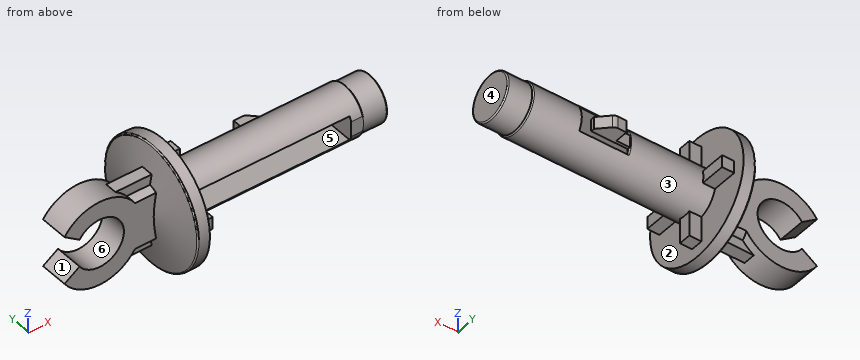
```python
from build123d import *

# Parameters (mm, degrees)
SCHIZZO1_R                    = 2
ESTRUSIONE_ESTRUSIONE1_DEPTH  = 17
SCHIZZO2_OUTSIDE_W            = 9.584
SCHIZZO2_OUTSIDE_H            = 9.584
SCHIZZO2_OUTSIDE_R            = 1.9
TAGLIO_ESTRUSIONE1_DEPTH      = 2
SCHIZZO6_W                    = 15
SCHIZZO6_H                    = 4
TAGLIO_ESTRUSIONE3_DEPTH      = 0.1
TAGLIO_ESTRUSIONE4_DEPTH      = 1.7
TAGLIO_ESTRUSIONE4_DEPTH_BACK = 18.23368794
SCHIZZO5_W                    = 13
SCHIZZO5_H                    = 2
SCHIZZO7_W                    = 4
SCHIZZO7_H                    = 2
TAGLIO_ESTRUSIONE5_DEPTH      = 18.555910686
ESTRUSIONE_ESTRUSIONE2_DEPTH  = 0.5
TAGLIO_ESTRUSIONE6_DEPTH      = 0.07
ESTRUSIONE_ESTRUSIONE4_DEPTH  = 0.5
ESTRUSIONE_ESTRUSIONE5_DEPTH  = 0.5
SCHIZZO20_R                   = 5
ESTRUSIONE_ESTRUSIONE6_DEPTH  = 1
SCHIZZO23_R                   = 2.25
ESTRUSIONE_ESTRUSIONE7_DEPTH  = 3
ESTRUSIONE_ESTRUSIONE10_DEPTH = 1.15
ESTRUSIONE_ESTRUSIONE8_DEPTH  = 0.5
SCHIZZO35_W                   = 3
SCHIZZO35_H                   = 3.867815922
TAGLIO_ESTRUSIONE7_DEPTH      = 1.3
RACCORDO22_R                  = 0.5
RACCORDO23_R                  = 0.1
RACCORDO24_R                  = 0.1
RACCORDO25_R                  = 0.1
RACCORDO28_R                  = 0.1


# Some blends are built 0.0001 mm under size
with BuildPart() as part:
    # Schizzo1 → Estrusione-Estrusione1 (new body)
    with BuildSketch(Plane(origin=(0, 0, 0), x_dir=(0, 0, -1), z_dir=(1, 0, 0))):
        Circle(SCHIZZO1_R)
    extrude(amount=-ESTRUSIONE_ESTRUSIONE1_DEPTH)

    # Schizzo2 outside → Taglio-Estrusione1 (cut)
    with BuildSketch(Plane(origin=(0, 0, 0), x_dir=(0, 0, -1), z_dir=(1, 0, 0))):
        Rectangle(SCHIZZO2_OUTSIDE_W, SCHIZZO2_OUTSIDE_H)
        Circle(SCHIZZO2_OUTSIDE_R, mode=Mode.SUBTRACT)
    extrude(amount=-TAGLIO_ESTRUSIONE1_DEPTH, mode=Mode.SUBTRACT)

    # Schizzo6 → Taglio-Estrusione3 (cut)
    with BuildSketch(Plane(origin=(0, -2, 0), x_dir=(-1, 0, 0), z_dir=(0, -1, 0))):
        with Locations((9.5, 0)):
            Rectangle(SCHIZZO6_W, SCHIZZO6_H)
    extrude(amount=-TAGLIO_ESTRUSIONE3_DEPTH, mode=Mode.SUBTRACT)

    # Schizzo5 → Taglio-Estrusione4 (cut, two sides: drawn at the far end of the back side and taken through both)
    with BuildSketch(Plane(origin=(0, 0, 0), x_dir=(1, 0, 0), z_dir=(0, 1, 0)).offset(-TAGLIO_ESTRUSIONE4_DEPTH_BACK)):
        with Locations((-9.5, 0)):
            Rectangle(SCHIZZO5_W, SCHIZZO5_H)
    extrude(amount=TAGLIO_ESTRUSIONE4_DEPTH + TAGLIO_ESTRUSIONE4_DEPTH_BACK, mode=Mode.SUBTRACT)

    # Schizzo7 → Taglio-Estrusione5 (cut, through all)
    with BuildSketch(Plane(origin=(0, 2, 0), x_dir=(1, 0, 0), z_dir=(0, 1, 0))):
        with Locations((-8, 0)):
            Rectangle(SCHIZZO7_W, SCHIZZO7_H)
    extrude(amount=-TAGLIO_ESTRUSIONE5_DEPTH, mode=Mode.SUBTRACT)

    # Schizzo12 → Estrusione-Estrusione2 (add, symmetric)
    with BuildSketch(Plane.XY):
        Polygon((-10, 2), (-8.9, 2), (-8.9, 3), (-8, 3), (-7, 2), (-7, 1.7), (-10, 1.7), align=None)
    extrude(amount=ESTRUSIONE_ESTRUSIONE2_DEPTH, both=True)

    # Schizzo16 → Taglio-Estrusione6 (cut)
    with BuildSketch(Plane(origin=(0, 2, 0), x_dir=(1, 0, 0), z_dir=(0, 1, 0))):
        Polygon((-8.9, 0.5), (-10, 0.5), (-10, 0), (-10, -0.5), (-8.9, -0.5), align=None)
    extrude(amount=-TAGLIO_ESTRUSIONE6_DEPTH, mode=Mode.SUBTRACT)

    # Schizzo17 → Estrusione-Estrusione4 (add, symmetric)
    with BuildSketch(Plane.XY):
        Polygon((-17, 4), (-16, 4), (-16, 0.047058824), (-17, 0.05), align=None)
    estrusione_estrusione4 = extrude(amount=ESTRUSIONE_ESTRUSIONE4_DEPTH, both=True)

    # Specchia2: Estrusione-Estrusione4 across plane
    add(estrusione_estrusione4.mirror(Plane.ZX))

    # Schizzo19 → Estrusione-Estrusione5 (add, symmetric)
    with BuildSketch(Plane(origin=(0, 0, 0), x_dir=(1, 0, 0), z_dir=(0, 1, 0))):
        Polygon((-17, 2), (-17, 0), (-16, 0), (-16, 2), (-16, 4), (-17, 4), align=None)
    estrusione_estrusione5 = extrude(amount=ESTRUSIONE_ESTRUSIONE5_DEPTH, both=True)

    # Specchia5: Estrusione-Estrusione5 across plane
    add(estrusione_estrusione5.mirror(Plane.XY))

    # Schizzo20 → Estrusione-Estrusione6 (add)
    with BuildSketch(Plane.ZY.offset(17)):
        Circle(SCHIZZO20_R)
    extrude(amount=ESTRUSIONE_ESTRUSIONE6_DEPTH)

    # Schizzo23 → Estrusione-Estrusione7 (add)
    with BuildSketch(Plane.ZY.offset(18)):
        Circle(SCHIZZO23_R)
    extrude(amount=ESTRUSIONE_ESTRUSIONE7_DEPTH)

    # Schizzo22 → Estrusione-Estrusione10 (add, symmetric)
    with BuildSketch(Plane(origin=(0, 0, 0), x_dir=(1, 0, 0), z_dir=(0, 1, 0))):
        with BuildLine():
            Line((-24.762298216, -1.129872594), (-26, -1.977277039))
            ThreePointArc((-26, -1.977277039), (-19.612029171, 0), (-26, 1.977277039))
            Line((-26, 1.977277039), (-24.762298216, 1.129872594))
            ThreePointArc((-24.762298216, 1.129872594), (-21.112029171, 0), (-24.762298216, -1.129872594))
        make_face()
    extrude(amount=ESTRUSIONE_ESTRUSIONE10_DEPTH, both=True)

    # Schizzo34 → Estrusione-Estrusione8 (add, symmetric)
    with BuildSketch(Plane(origin=(0, 0, 0), x_dir=(1, 0, 0), z_dir=(0, 1, 0))):
        Polygon((-18, 3), (-21.309253533, 3), (-18, 0), align=None)
    estrusione_estrusione8 = extrude(amount=ESTRUSIONE_ESTRUSIONE8_DEPTH, both=True)

    # Specchia6: Estrusione-Estrusione8 across plane
    add(estrusione_estrusione8.mirror(Plane.XY))

    # Schizzo35 → Taglio-Estrusione7 (cut)
    with BuildSketch(Plane(origin=(0, 1.15, 0), x_dir=(1, 0, 0), z_dir=(0, 1, 0))):
        with Locations((-19.5, 0)):
            Rectangle(SCHIZZO35_W, SCHIZZO35_H)
    taglio_estrusione7 = extrude(amount=TAGLIO_ESTRUSIONE7_DEPTH, mode=Mode.SUBTRACT)

    # Specchia7: Taglio-Estrusione7 across plane
    add(taglio_estrusione7.mirror(Plane.ZX), mode=Mode.SUBTRACT)

    # Raccordo22
    raccordo22_edges = [part.edges().sort_by_distance(p)[0] for p in [
        (-8, 3, 0),
    ]]
    fillet(raccordo22_edges, radius=RACCORDO22_R)

    # Raccordo23
    raccordo23_edges = [part.edges().sort_by_distance(p)[0] for p in [
        (-2, 2, 0),
    ]]
    fillet(raccordo23_edges, radius=RACCORDO23_R - 0.0001)  # a hair under: the kernel refuses the full size

    # Raccordo24
    raccordo24_edges = [part.edges().sort_by_distance(p)[0] for p in [
        (0, 0, 1.9),
    ]]
    fillet(raccordo24_edges, radius=RACCORDO24_R)

    # Raccordo25
    raccordo25_edges = [part.edges().sort_by_distance(p)[0] for p in [
        (-18, 0, -5),
    ]]
    fillet(raccordo25_edges, radius=RACCORDO25_R)

    # Raccordo28
    # the kernel refuses this fillet: 0.1 mm, written as the material it takes off along each edge
    with BuildSketch(Plane(origin=(-10, 0, 0), x_dir=(0, 0.7969175395012055, 0.6040881022130338), z_dir=(0, -0.6040881022130338, 0.7969175395012055))) as raccordo28_piece_1_section:
        with BuildLine():
            CenterArc((2 - RACCORDO28_R, RACCORDO28_R), RACCORDO28_R, 270, 90)
            Line((2 - RACCORDO28_R, 0), (2, 0))
            Line((2, 0), (2, RACCORDO28_R))
        make_face()
    raccordo28_piece_1 = revolve(axis=Axis((-10, 0, 0), (-1, 0, 0)), revolution_arc=74.326501832, mode=Mode.PRIVATE)
    raccordo28_piece_1 = split(raccordo28_piece_1, bisect_by=Plane(origin=(-10.022414525, 1.819827674, 1), z_dir=(0, 0, -1)), keep=Keep.TOP, mode=Mode.PRIVATE)
    raccordo28_piece_1 = split(raccordo28_piece_1, bisect_by=Plane(origin=(-10.022414525, 1.819827674, 0.5), z_dir=(0, 0, 1)), keep=Keep.TOP, mode=Mode.PRIVATE)
    raccordo28_piece_1 = split(raccordo28_piece_1, bisect_by=Plane(origin=(-10.022414525, 1.93, 0.756995565), z_dir=(0, -1, 0)), keep=Keep.TOP, mode=Mode.PRIVATE)
    add(raccordo28_piece_1, mode=Mode.SUBTRACT)
    with BuildSketch(Plane(origin=(-10, 0, 0), x_dir=(0, 0.7969175395012055, 0.6040881022130338), z_dir=(0, -0.6040881022130338, 0.7969175395012055))) as raccordo28_piece_2_section:
        with BuildLine():
            CenterArc((2 - RACCORDO28_R, RACCORDO28_R), RACCORDO28_R, 270, 90)
            Line((2 - RACCORDO28_R, 0), (2, 0))
            Line((2, 0), (2, RACCORDO28_R))
        make_face()
    raccordo28_piece_2 = revolve(axis=Axis((-10, 0, 0), (-1, 0, 0)), revolution_arc=74.326501832, mode=Mode.PRIVATE)
    raccordo28_piece_2 = split(raccordo28_piece_2, bisect_by=Plane(origin=(-10.044225117, 1.932988234, 0.5), z_dir=(0, 0, 1)), keep=Keep.TOP, mode=Mode.PRIVATE)
    raccordo28_piece_2 = split(raccordo28_piece_2, bisect_by=Plane(origin=(-10.044225117, 1.93, 0.511192028), z_dir=(0, 1, 0)), keep=Keep.TOP, mode=Mode.PRIVATE)
    add(raccordo28_piece_2, mode=Mode.SUBTRACT)
    with BuildSketch(Plane(origin=(-10, 0, 0), x_dir=(0, 0.7969175395012055, 0.6040881022130338), z_dir=(0, -0.6040881022130338, 0.7969175395012055))) as raccordo28_piece_3_section:
        with BuildLine():
            CenterArc((2 - RACCORDO28_R, RACCORDO28_R), RACCORDO28_R, 270, 90)
            Line((2 - RACCORDO28_R, 0), (2, 0))
            Line((2, 0), (2, RACCORDO28_R))
        make_face()
    raccordo28_piece_3 = revolve(axis=Axis((-10, 0, 0), (-1, 0, 0)), revolution_arc=74.326501832, mode=Mode.PRIVATE)
    raccordo28_piece_3 = split(raccordo28_piece_3, bisect_by=Plane(origin=(-10.022414524, 1.819827674, -1), z_dir=(0, 0, 1)), keep=Keep.TOP, mode=Mode.PRIVATE)
    raccordo28_piece_3 = split(raccordo28_piece_3, bisect_by=Plane(origin=(-10.022414524, 1.93, -0.756995565), z_dir=(0, -1, 0)), keep=Keep.TOP, mode=Mode.PRIVATE)
    raccordo28_piece_3 = split(raccordo28_piece_3, bisect_by=Plane(origin=(-10.022414524, 1.819827674, -0.5), z_dir=(0, 0, -1)), keep=Keep.TOP, mode=Mode.PRIVATE)
    add(raccordo28_piece_3, mode=Mode.SUBTRACT)
    with BuildSketch(Plane(origin=(-10, 0, 0), x_dir=(0, 0.7969175395012055, 0.6040881022130338), z_dir=(0, -0.6040881022130338, 0.7969175395012055))) as raccordo28_piece_4_section:
        with BuildLine():
            CenterArc((2 - RACCORDO28_R, RACCORDO28_R), RACCORDO28_R, 270, 90)
            Line((2 - RACCORDO28_R, 0), (2, 0))
            Line((2, 0), (2, RACCORDO28_R))
        make_face()
    raccordo28_piece_4 = revolve(axis=Axis((-10, 0, 0), (-1, 0, 0)), revolution_arc=74.326501832, mode=Mode.PRIVATE)
    raccordo28_piece_4 = split(raccordo28_piece_4, bisect_by=Plane(origin=(-10.040080162, 1.981654904, 0.5), z_dir=(0, 0, -1)), keep=Keep.TOP, mode=Mode.PRIVATE)
    raccordo28_piece_4 = split(raccordo28_piece_4, bisect_by=Plane(origin=(-10.040080162, 1.93, 0), z_dir=(0, 1, 0)), keep=Keep.TOP, mode=Mode.PRIVATE)
    raccordo28_piece_4 = split(raccordo28_piece_4, bisect_by=Plane(origin=(-10.040080162, 1.981654904, -0.5), z_dir=(0, 0, 1)), keep=Keep.TOP, mode=Mode.PRIVATE)
    add(raccordo28_piece_4, mode=Mode.SUBTRACT)
    with BuildSketch(Plane(origin=(-10, 0, 0), x_dir=(0, 0.7969175395012055, 0.6040881022130338), z_dir=(0, -0.6040881022130338, 0.7969175395012055))) as raccordo28_piece_5_section:
        with BuildLine():
            CenterArc((2 - RACCORDO28_R, RACCORDO28_R), RACCORDO28_R, 270, 90)
            Line((2 - RACCORDO28_R, 0), (2, 0))
            Line((2, 0), (2, RACCORDO28_R))
        make_face()
    raccordo28_piece_5 = revolve(axis=Axis((-10, 0, 0), (-1, 0, 0)), revolution_arc=74.326501832, mode=Mode.PRIVATE)
    raccordo28_piece_5 = split(raccordo28_piece_5, bisect_by=Plane(origin=(-10.044225117, 1.93, -0.511192028), z_dir=(0, 1, 0)), keep=Keep.TOP, mode=Mode.PRIVATE)
    raccordo28_piece_5 = split(raccordo28_piece_5, bisect_by=Plane(origin=(-10.044225117, 1.932988234, -0.5), z_dir=(0, 0, -1)), keep=Keep.TOP, mode=Mode.PRIVATE)
    add(raccordo28_piece_5, mode=Mode.SUBTRACT)

    # Estrusione-Estrusione9 cone 1 section (through the dimple's axis) → Estrusione-Estrusione9 (revolve)
    with BuildSketch(Plane(origin=(-18, 0, 0), x_dir=(0, 0, -1), z_dir=(0, 1, 0))):
        Polygon((0, 0), (4.9, 0), (0, 0.864002205), align=None)
    revolve(axis=Axis((-18, 0, 0), (-1, 0, 0)))


solid = part.part
```
Part model, mm, in its own coordinate system. Face numbers are marked on the shaded views. A direction names the side the tool comes from. Round coordinates to 2 decimals unless told otherwise and drop trailing zeros. Write each loop counter-clockwise with the first axis right and the second up, starting at its lowest first coordinate (ties: lowest second). Pieces come first, ordered by that corner, then holes. Notation, with made-up numbers: (13, 6.25) -> (72, 6.25) arc R6 cw to (72, 10.25) -> close; hole circle Ø8 at (78, 89). An arc over 180 degrees is marked (long way). Return JSON: item names as keys, results as strings. Group by question number.
Q1. Which spindle directions (+Z, -Z, +X, -X, +Y, -Y) get a long thin tool onto all of the face, cutting with end or side? Do the marked faces 1 and 2. Say none if no direction does.
Q2. Pin check, flat tips, straight feed: pin 1 (5 mm diameter, centred on x = -23.11, z = 0, fed in from -Y); pin 2 (1.6 mm diameter, centred on y = -1, z = 0, fed in from -X); pin 3 (0.9 mm diameter, centred on x = -20, z = 2.5, fed in from -Y). Stop position of each tip, or through.
Q3. Probe L1, parallel to Z at x = -15, y = 1; L2, parallel to Z at x = -17.5, y = -3; L3, parallel to X at y = 1.5, z = -0.75. List the from-to ranges inside material, lowest first. Write a range as [from, to].
Q4. Mould opens along Z. For the marked faces 3, 4, 5 and 6 say: pulls with the +Z half, pulls with the -Z half, needs draft (parallel to the pull), parting line crosses it, or undercut.
Q5. Saw through at C-C on x = -4.5. Write the cut outline in (y, z).
Q6. Saw through at A-A on x = -22.5. Write the cut outline in (y, z).
Answer:
{
 "1": {"face 1": "-X, +Y, -Y", "face 2": "+X"},
 "2": {"pin 1": "y = -1.15", "pin 2": "x = -21.28", "pin 3": "y = -0.93"},
 "3": {"L1": "[-1.73, -1], [1, 1.73]", "L2": "[-4, 4]", "L3": "[-18.57, -16], [-3, 0]"},
 "4": {"face 3": "parting line crosses it", "face 4": "needs draft", "face 5": "undercut", "face 6": "undercut"},
 "5": {"outline": "(-1.73, -1) arc R2 ccw (long way) to (-1.73, 1) -> (1.7, 1) -> (1.7, -1) -> close"},
 "6": {"outline": "(-1.15, -3.45) -> (1.15, -3.45) -> (1.15, -1.9) -> (-1.15, -1.9) -> close; (-1.15, 1.9) -> (1.15, 1.9) -> (1.15, 3.45) -> (-1.15, 3.45) -> close"}
}
